```python
from build123d import *

# Parameters (mm, degrees)
SKETCH1_R           = 1.5
BOSS_EXTRUDE1_DEPTH = 3


with BuildPart() as part:
    # Sketch1 → Boss-Extrude1 (new body)
    with BuildSketch(Plane(origin=(0, 0, 0), x_dir=(1, 0, 0), z_dir=(0, 1, 0))):
        with BuildLine():
            Line((72, 15), (-72, 15))
            ThreePointArc((-72, 15), (-74.121320344, 14.121320344), (-75, 12))
            Line((-75, 12), (-75, -12))
            ThreePointArc((-75, -12), (-74.121320344, -14.121320344), (-72, -15))
            Line((-72, -15), (72, -15))
            ThreePointArc((72, -15), (74.121320344, -14.121320344), (75, -12))
            Line((75, -12), (75, 12))
            ThreePointArc((75, 12), (74.121320344, 14.121320344), (72, 15))
        make_face()
        with Locations((65, 0)):
            Circle(SKETCH1_R, mode=Mode.SUBTRACT)
        with Locations((-65, 0)):
            Circle(SKETCH1_R, mode=Mode.SUBTRACT)
        with BuildLine():
            Line((51.5, -7.5), (48.5, -7.5))
            ThreePointArc((48.5, -7.5), (47.792893219, -7.207106781), (47.5, -6.5))
            Line((47.5, -6.5), (47.5, 6.5))
            ThreePointArc((47.5, 6.5), (47.792893219, 7.207106781), (48.5, 7.5))
            Line((48.5, 7.5), (51.5, 7.5))
            ThreePointArc((51.5, 7.5), (52.207106781, 7.207106781), (52.5, 6.5))
            Line((52.5, 6.5), (52.5, -6.5))
            ThreePointArc((52.5, -6.5), (52.207106781, -7.207106781), (51.5, -7.5))
        make_face(mode=Mode.SUBTRACT)
        with BuildLine():
            Line((-47.5, -6.5), (-47.5, 6.5))
            ThreePointArc((-47.5, 6.5), (-47.792893219, 7.207106781), (-48.5, 7.5))
            Line((-48.5, 7.5), (-51.5, 7.5))
            ThreePointArc((-51.5, 7.5), (-52.207106781, 7.207106781), (-52.5, 6.5))
            Line((-52.5, 6.5), (-52.5, -6.5))
            ThreePointArc((-52.5, -6.5), (-52.207106781, -7.207106781), (-51.5, -7.5))
            Line((-51.5, -7.5), (-48.5, -7.5))
            ThreePointArc((-48.5, -7.5), (-47.792893219, -7.207106781), (-47.5, -6.5))
        make_face(mode=Mode.SUBTRACT)
    extrude(amount=BOSS_EXTRUDE1_DEPTH)


solid = part.part
```
Geometry check sheet. Reference: the model listing, model coordinates, mm. A direction names the side the tool comes from. Coordinates: 2 decimals unless noted, no trailing zeros. Loops run counter-clockwise (first coordinate to the right, second up) from the corner with the lowest first, then second, coordinate; pieces in that order, holes last. Notation, with made-up numbers: (37.5, 60.5) -> (77.5, 60.5) arc R24 cw to (77.5, 89.5) -> close; hole circle Ø4 at (22.5, -30.75). An arc over 180 degrees is marked (long way). Put each result on its own line as item: value.
1) Gauge pin test, flat end, axial feed: pin 1 Ø4 at (x, z) = (65, 0) entering from +Y. Record the tip position at first contact, or that the pin passes through.
Result set:
pin 1: stops at y = 3
2) Thickness scan on line 1 (X direction, y = 0.35, z = -4.5); line 2 (X direction, y = 1.1, z = 0); line 3 (Z direction, x = 65, y = 1.45). Record the ranges inside material, lowest first.
Result set:
line 1: x = -75 to -52.5, -47.5 to 47.5, 52.5 to 75
line 2: x = -75 to -66.5, -63.5 to -52.5, -47.5 to 47.5, 52.5 to 63.5, 66.5 to 75
line 3: z = -15 to -1.5, 1.5 to 15
3) Cross-section at C-C on y = 1.05. Record the boundary of the cut face in (x, z), plus the area to 3 significant figures.
Result set:
outline: (-75, -12) arc R3 ccw to (-72, -15) -> (72, -15) arc R3 ccw to (75, -12) -> (75, 12) arc R3 ccw to (72, 15) -> (-72, 15) arc R3 ccw to (-75, 12) -> close; hole circle Ø3 at (-65, 0); hole (-52.5, -6.5) arc R1 ccw to (-51.5, -7.5) -> (-48.5, -7.5) arc R1 ccw to (-47.5, -6.5) -> (-47.5, 6.5) arc R1 ccw to (-48.5, 7.5) -> (-51.5, 7.5) arc R1 ccw to (-52.5, 6.5) -> close; hole (47.5, -6.5) arc R1 ccw to (48.5, -7.5) -> (51.5, -7.5) arc R1 ccw to (52.5, -6.5) -> (52.5, 6.5) arc R1 ccw to (51.5, 7.5) -> (48.5, 7.5) arc R1 ccw to (47.5, 6.5) -> close; hole circle Ø3 at (65, 0)
area: 4,330 mm^2
4) Cross-section at A-A on x = 65. Record the boundary of the cut face in (y, z), plus the area to 3 significant figures.
Result set:
outline: (0, -15) -> (3, -15) -> (3, -1.5) -> (0, -1.5) -> close; (0, 1.5) -> (3, 1.5) -> (3, 15) -> (0, 15) -> close
area: 81.0 mm^2
5) Cross-section at B-B on z = 0. Record the boundary of the cut face in (x, y).
Result set:
outline: (-75, 0) -> (-66.5, 0) -> (-66.5, 3) -> (-75, 3) -> close; (-63.5, 0) -> (-52.5, 0) -> (-52.5, 3) -> (-63.5, 3) -> close; (-47.5, 0) -> (47.5, 0) -> (47.5, 3) -> (-47.5, 3) -> close; (52.5, 0) -> (63.5, 0) -> (63.5, 3) -> (52.5, 3) -> close; (66.5, 0) -> (75, 0) -> (75, 3) -> (66.5, 3) -> close
6) Release check for a two-part mould opening along X. For faces 3 (the cylindrical face through (-74.1, 1.48, -14.14)), 4 (the flat face through (-52.5, 1, 0)), 5 (the flat face through (1, 1, -15)) record: released by +X, released by -X, zero draft, split by the parting line, or undercut.
Result set:
face 3: released by -X
face 4: undercut
face 5: zero draft
7) Tool access check on faces 1 (the flat face through (-1, 1, 15)), 2 (the flat face through (52.5, 1, 0)). Record the directions out of +Z, -Z, +X, -X, +Y, -Y that give a thin tool (end or side, any length) a straight path to the whole face; none if there is none.
Result set:
face 1: +Z, +X, -X, +Y, -Y
face 2: +Y, -Y
